Verification items for the finished model (mm, model axes). Face numbers are marked on the shaded views. Give positions to 0.01 mm unless a question says otherwise; leave off trailing zeros. Use one line per item in the form item = value. Start each with the question number.
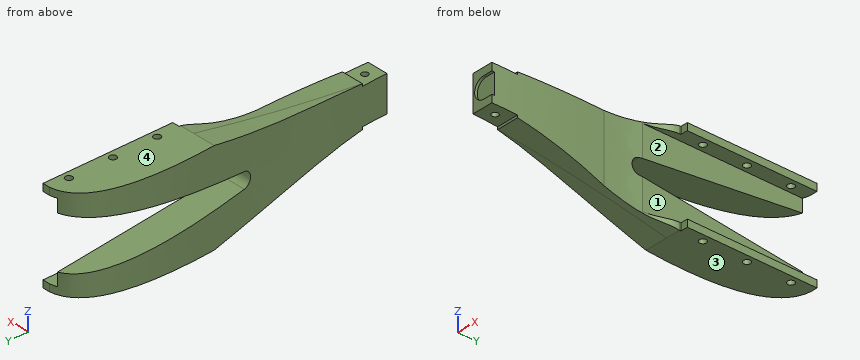
from build123d import *

# Parameters (mm, degrees)
BOSS_EXTRUDE2_DEPTH        = 35.5
CUT_EXTRUDE1_DEPTH         = 17.75
CUT_EXTRUDE2_DEPTH         = 2.8
SKETCH5_W                  = 2.8
SKETCH5_H                  = 2.75
BOSS_EXTRUDE3_DEPTH        = 50
CUT_EXTRUDE3_DEPTH         = 15
F_2_7_2_7_DIAMETER_HOLE1_D = 2.7
M3_TAPPED_HOLE1_D          = 2.5
CUT_EXTRUDE4_DEPTH         = 126.902937834
CUT_EXTRUDE4_DEPTH_BACK    = 126.902937834
SKETCH12_W                 = 1.496855304
SKETCH12_H                 = 10
SKETCH12_W_2               = 1.571931937
CUT_EXTRUDE5_DEPTH         = 20
CUT_EXTRUDE6_DEPTH         = 1


with BuildPart() as part:
    # Sketch1 → Boss-Extrude2 (new body)
    with BuildSketch(Plane.XY):
        with BuildLine():
            Line((5.6, 35.6), (5.6, -15))
            add(Edge.make_bspline(
                [(5.6, -15), (5.6, -17.274393969), (1.604195195, -25.847964508), (2.415841027, -35.113621235), (3.409417942, -42.11611418)],
                knots=[0, 0, 0, 0, 0.227789152, 0.921500182, 0.921500182, 0.921500182, 0.921500182], degree=3))
            add(Edge.make_bspline(
                [(3.409417942, -42.11611418), (14.021423643, -91.198515752), (3.540705721, -122.805120936)],
                knots=[0, 0, 0, 1, 1, 1], degree=2))
            Line((3.540705721, -122.805120936), (-4.088116427, -120.408076375))
            add(Edge.make_bspline(
                [(5.6, 35.6), (-12.367874994, 33.521263174), (-8.7823866, -50.782642202), (5.954211422, -91.451497422), (-4.088116427, -120.408076375)],
                knots=[0, 0, 0, 0, 0.40530679, 1, 1, 1, 1], degree=3))
        make_face()
    extrude(amount=BOSS_EXTRUDE2_DEPTH)

    # Sketch3 → Cut-Extrude1 (cut, symmetric)
    with BuildSketch(Plane(origin=(0, 0, 0), x_dir=(0, 0, -1), z_dir=(1, 0, 0))):
        with BuildLine():
            Line((0, -14.98237842), (29.62736343, -14.98237842))
            Line((29.62736343, -14.98237842), (29.62736343, -131.572481325))
            Line((29.62736343, -131.572481325), (-60.547074518, -131.572481325))
            Line((-60.547074518, -131.572481325), (-60.547074518, -14.98237842))
            Line((-60.547074518, -14.98237842), (-35.5, -14.98237842))
            add(Edge.make_bspline(
                [(-35.5, -14.98237842), (-28.308780975, -49.75857776), (-24.077993602, -85.166412163), (-22.769212626, -120.408076375)],
                knots=[0, 0, 0, 0, 1, 1, 1, 1], degree=3))
            Line((-22.769212626, -120.408076375), (-12.75, -120.408076375))
            add(Edge.make_bspline(
                [(0, -14.98237842), (-7.191219025, -49.75857776), (-11.441219025, -85.166412163), (-12.75, -120.408076375)],
                knots=[0, 0, 0, 0, 1, 1, 1, 1], degree=3))
        make_face()
    extrude(amount=CUT_EXTRUDE1_DEPTH, both=True, mode=Mode.SUBTRACT)

    # Sketch4 → Cut-Extrude2 (cut)
    with BuildSketch(Plane(origin=(5.6, 0, 0), x_dir=(0, 0, -1), z_dir=(1, 0, 0))):
        Polygon((-2.75, 35.6), (-32.75, 35.6), (-32.75, -15.000000007), (-32.75, -32.018147114), (-2.75, -32.018147114), (-2.75, -15.000000007), align=None)
    extrude(amount=-CUT_EXTRUDE2_DEPTH, mode=Mode.SUBTRACT)

    # Sketch5 → Boss-Extrude3 (add)
    with BuildSketch(Plane(origin=(0, 35.6, 0), x_dir=(1, 0, 0), z_dir=(0, 1, 0))):
        with Locations((7, -1.375)):
            Rectangle(SKETCH5_W, SKETCH5_H)
        with Locations((7, -34.125)):
            Rectangle(SKETCH5_W, SKETCH5_H)
    extrude(amount=-BOSS_EXTRUDE3_DEPTH)

    # Sketch6 → Cut-Extrude3 (cut, symmetric)
    with BuildSketch(Plane(origin=(0, 0, 0), x_dir=(0, 0, -1), z_dir=(1, 0, 0))):
        with BuildLine():
            Line((-7.75, 34.96933844), (-14.781773193, -27.808788024))
            ThreePointArc((-14.781773193, -27.808788024), (-17.763748777, -30.474846509), (-20.744622729, -27.807556366))
            Line((-20.744622729, -27.807556366), (-27.75, 34.96933844))
            Line((-27.75, 34.96933844), (-7.75, 34.96933844))
        make_face()
    extrude(amount=CUT_EXTRUDE3_DEPTH, both=True, mode=Mode.SUBTRACT)

    # Ø2.7 (2.7) Diameter Hole1 (through all)
    with Locations(Plane.XY.offset(35.5)):
        with Locations((5.6, 28.1), (5.6, 11.1), (5.6, -5.9)):
            Hole(F_2_7_2_7_DIAMETER_HOLE1_D / 2)

    # M3 Tapped Hole1 (through all)
    with Locations(Plane.XY.offset(35.5)):
        with Locations((4.5, -85)):
            Hole(M3_TAPPED_HOLE1_D / 2)

    # Sketch12 → Cut-Extrude4 (cut, two sides: drawn at the far end of the back side and taken through both)
    with BuildSketch(Plane(origin=(0, 0, 0), x_dir=(0, 0, -1), z_dir=(1, 0, 0)).offset(-CUT_EXTRUDE4_DEPTH_BACK)):
        with Locations((-10.144277768, -85)):
            Rectangle(SKETCH12_W, SKETCH12_H)
        with Locations((-25.408624424, -85)):
            Rectangle(SKETCH12_W_2, SKETCH12_H)
    extrude(amount=CUT_EXTRUDE4_DEPTH + CUT_EXTRUDE4_DEPTH_BACK, mode=Mode.SUBTRACT)

    # Sketch14 → Cut-Extrude5 (cut)
    with BuildSketch(Plane(origin=(0, 0, 10.89270542), x_dir=(-1, 0, 0), z_dir=(0, 0, -1))):
        Polygon((-8.720315384, -90), (6.272671273, -90), (6.272671273, -124.093634091), (-10.541100015, -124.093634091), (-10.541100015, -90), align=None)
    extrude(amount=-CUT_EXTRUDE5_DEPTH, mode=Mode.SUBTRACT)

    # Sketch15 → Cut-Extrude6 (cut)
    with BuildSketch(Plane(origin=(0, -90, 0), x_dir=(-1, 0, 0), z_dir=(0, -1, 0))):
        with BuildLine():
            Line((-5.220315384, -13.74270542), (-8.720315384, -13.74270542))
            Line((-8.720315384, -13.74270542), (-9.623354914, -13.74270542))
            Line((-9.623354914, -13.74270542), (-9.623354914, -21.74270542))
            Line((-9.623354914, -21.74270542), (-5.220315384, -21.74270542))
            ThreePointArc((-5.220315384, -21.74270542), (-1.220315384, -17.74270542), (-5.220315384, -13.74270542))
        make_face()
    extrude(amount=-CUT_EXTRUDE6_DEPTH, mode=Mode.SUBTRACT)


solid = part.part
Item 1: Material ranges on line 1 (Z direction, x = 5, y = -14.5); line 2 (X direction, y = -85, z = 14.25); line 3 (Z direction, x = -2.25, y = 28.5), recorded low to high.
Item 2: Gauge pin test, flat ends, axial feed: pin 1 Ø2.5 at (x, y) = (4, -84) entering from +Z; pin 2 Ø0.5 at (y, z) = (-15, 2) entering from +X; pin 3 Ø3 at (x, y) = (-2.5, -62) entering from +Z; pin 4 Ø2 at (x, y) = (5, -6.5) entering from +Z. Record the tip position at first contact, or that the pin passes through.
Item 3: Sectioned sample at A-A, the plane y = 28.1. State how many separate pieces and enclosed holes the cut face has, and give its area (3 significant figures).
Item 4: Draft check along Z on the marked faces 1, 2, 3 and 4. Enter one of: +Z half, -Z half, draft (parallel to the pull), parting line (faces both ways), or undercut.
Outcome:
q1.line_1 = 0 to 2.75, 32.75 to 35.5
q1.line_2 = 0.3 to 3.25, 5.75 to 8.73
q1.line_3 = 0 to 8.47, 27.03 to 35.5
q2.pin_1 = 24.62
q2.pin_2 = 5.6
q2.pin_3 = 27.81
q2.pin_4 = 35.5
q3.separate_pieces = 4
q3.enclosed_holes = 0
q3.area = 146 mm^2
q4.face_1 = undercut
q4.face_2 = undercut
q4.face_3 = -Z half
q4.face_4 = +Z half
